Read the model definition and answer for the solid it produces. Units are mm, in the model's axes. Coordinates: 2 decimals unless noted, no trailing zeros. Write each loop counter-clockwise with the first axis right and the second up, starting at its lowest first coordinate (ties: lowest second). Pieces come first, ordered by that corner, then holes. Notation, with made-up numbers: (33, 74) -> (61, 74) arc R20 cw to (61, 110) -> close; hole circle Ø8 at (27, 32.5). An arc over 180 degrees is marked (long way). Write item = value, one per line. Start each with the question number.
1) Section A-A (y = -2) is taken. Determine the outline of the cut face in (x, z), plus the area to 3 significant figures.
2) Flat-ended cylindrical pins translate along their axes: pin 1 Ø3 at (x, y) = (134, -11) entering from -Z; pin 2 Ø0.9 at (x, z) = (77, 1.5) entering from -Y; pin 3 Ø1 at (y, z) = (-6.5, 1.5) entering from -X; pin 4 Ø1.5 at (y, z) = (-21.5, 1) entering from +X. Find the tip coordinate at first contact, or state that the pin passes through.
3) Find the intervals of material crossed by line 1 along Y through (x, z) = (77.5, 1.7); line 2 along X through (y, z) = (-12.75, 1.55), in increasing order. Write a range as from..to.
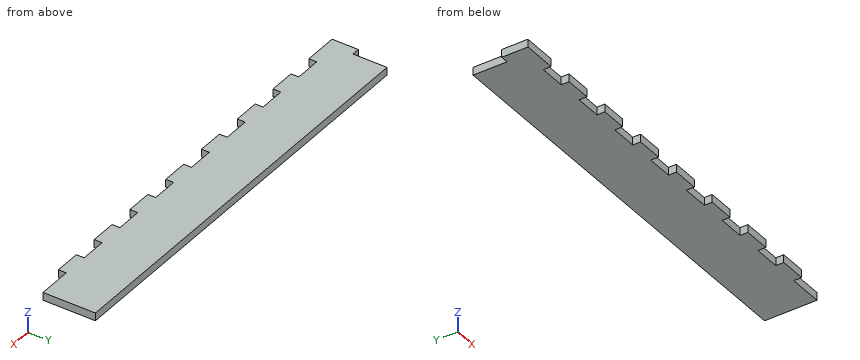
from build123d import *

# Parameters (mm, degrees)
ESQUISSE1_W                = 163
ESQUISSE1_H                = 20
BOSS_EXTRU_1_DEPTH         = 3
ESQUISSE2_W                = 10
ESQUISSE2_H                = 3
BOSS_EXTRU_2_DEPTH         = 3
R_P_TITION_LIN_AIRE1_COUNT = 8
R_P_TITION_LIN_AIRE1_PITCH = 20
ESQUISSE3_W                = 3
ESQUISSE3_H                = 10
BOSS_EXTRU_3_DEPTH         = 3


with BuildPart() as part:
    # Esquisse1 → Boss.-Extru.1 (new body)
    with BuildSketch(Plane.XY):
        with Locations((81.5, -10)):
            Rectangle(ESQUISSE1_W, ESQUISSE1_H)
    extrude(amount=BOSS_EXTRU_1_DEPTH)

    # Esquisse2 → Boss.-Extru.2 (add)
    with BuildSketch(Plane.XZ.offset(20)):
        with Locations((5, 1.5)):
            Rectangle(ESQUISSE2_W, ESQUISSE2_H)
    boss_extru_2 = extrude(amount=BOSS_EXTRU_2_DEPTH)

    # Répétition linéaire1: Boss.-Extru.2 ×8
    with Locations(*[(i * R_P_TITION_LIN_AIRE1_PITCH, 0, 0) for i in range(1, R_P_TITION_LIN_AIRE1_COUNT)]):
        add(boss_extru_2)

    # Esquisse3 → Boss.-Extru.3 (add)
    with BuildSketch(Plane.ZY):
        with Locations((1.5, -18)):
            Rectangle(ESQUISSE3_W, ESQUISSE3_H)
    extrude(amount=BOSS_EXTRU_3_DEPTH)


solid = part.part
Answer key:
q1.outline = (0, 0) -> (163, 0) -> (163, 3) -> (0, 3) -> close
q1.area = 489 mm^2
q2.pin_1 = 0
q2.pin_2 = -20
q2.pin_3 = 0
q2.pin_4 = 150
q3.line_1 = -20..0
q3.line_2 = 0..163
